from build123d import *

# Parameters (mm, degrees)
TROU_TARAUD_G1_161_D = 10.5


with BuildPart() as part:
    # Esquisse2 → Révolution1 (revolve)
    with BuildSketch(Plane.XY):
        Polygon((-19, 19.83574186), (-19, 4.75482653), (-3, 4.75482653), (-3, 3.289391775), (-3, -12.457506315), (0, -12.457506315), (0, -14.457506315), (-4.744922372, -14.457506315), (-7, -14.457506315), (-7, 2.75482653), (-9.300232951, 2.75482653), (-21, 2.75482653), (-21, 19.83574186), align=None)
    revolve(axis=Axis((0, 8.523766276, 0), (0, -1, 0)))

    # Trou taraudé G1/161 (through all)
    with Locations(Plane(origin=(1.240708844, -5.954064023, -6.889168423), x_dir=(-0.984166917609, 0, -0.17724412059), z_dir=(0.17724412059, 0, -0.984166917609))):
        with Locations((0, 0)):
            Hole(TROU_TARAUD_G1_161_D / 2)


solid = part.part
Geometry check sheet. Reference: the model listing, model coordinates, mm. A direction names the side the tool comes from. Give positions to 0.01 mm unless a question says otherwise; leave off trailing zeros. Loops run counter-clockwise (first coordinate to the right, second up) from the corner with the lowest first, then second, coordinate; pieces in that order, holes last. Notation, with made-up numbers: M -39.75,12 L -25.75,12 A26 ccw -25.75,46 Z; hole C 63.25,-31 d5. An arc over 180 degrees is marked long. Write each question's results on one line, items separated by ' | '.
1) Release check for a two-part mould opening along Y. For faces 1 (the face through (-9, 2.755, 0)), 2 (the face through (4.911, -4.377, 0.984)), 3 (the face through (0, 4.755, 4)) record: +Y half, -Y half, draft (parallel to the pull), parting line (faces both ways), or undercut.
Answers follow:
face 1: -Y half | face 2: undercut | face 3: +Y half
2) Section check B-B, the plane y = -5. Record the boundary of the cut face in (x, z), plus the area to 3 significant figures.
Answers follow:
outline: M -5.92,3.74 A7 ccw -4.24,-5.57 Z; M 4.24,5.57 L 5.92,-3.74 A7 ccw Z | area: 23.8 mm2
3) Section check C-C, the plane z = 14.5. Record the boundary of the cut face in (x, y), plus the area to 3 significant figures.
Answers follow:
outline: M -15.19,2.75 L 15.19,2.75 L 15.19,19.84 L 12.28,19.84 L 12.28,4.75 L -12.28,4.75 L -12.28,19.84 L -15.19,19.84 Z | area: 149 mm2
4) Section check D-D, the plane x = -1. Count the separate pieces of the cut face and the enclosed holes in it, plus the area to 3 significant figures.
Answers follow:
separate pieces: 3 | enclosed holes: 0 | area: 202 mm2
5) Gauge pin test, flat ends, axial feed: pin 1 (2 mm diameter, centred on x = -3.5, y = 9, fed in from -Z); pin 2 (1.8 mm diameter, centred on x = 1, z = -0.5, fed in from +Y); pin 3 (10 mm diameter, centred on y = -8, z = -9, fed in from +X). Record the tip position at first contact, or that the pin passes through.
Answers follow:
pin 1: z = -20.85 | pin 2: y = -12.46 | pin 3: x = 5.74
6) Tool access check on faces 4 (the face through (0, -14.458, 0)), 5 (the face through (0.65, 1.6, 2.93)), 6 (the face through (-6.466, -5.731, 2.681)). Record the directions out of +Z, -Z, +X, -X, +Y, -Y that give a thin tool (end or side, any length) a straight path to the whole face; none if there is none.
Answers follow:
face 4: +Z, -Z, +X, -X, -Y | face 5: +Y | face 6: -Y
7) Thickness scan on line 1 (X direction, y = 3, z = 0); line 2 (X direction, y = 16, z = 0). Record the ranges inside material, lowest first.
Answers follow:
line 1: -21 to -3, 3 to 21 | line 2: -21 to -19, 19 to 21
8) Section check A-A, the plane x = 13.5. Record the boundary of the cut face in (y, z), plus the area to 3 significant figures.
Answers follow:
outline: M 2.75,-16.09 L 19.84,-16.09 L 19.84,-13.37 L 4.75,-13.37 L 4.75,13.37 L 19.84,13.37 L 19.84,16.09 L 2.75,16.09 Z | area: 146 mm2
